from build123d import *

# Parameters (mm, degrees)
F0_R     = 17
F0_R_2   = 1.5
F0_R_3   = 1
F1_DEPTH = 15
F2_START = 10
F2_DEPTH = 15
F3_DEPTH = 5


# Not quite as in the source:
# - a feature names something its author has since deleted; it is built from what else it names


with BuildPart() as f1:
    # F0 (on Front) → F1 (new body)
    with BuildSketch(Plane.XZ):
        Circle(F0_R)
        with BuildLine():
            ThreePointArc((-4.2152867015, -5.2422664968), (-4.1715341961, -5.447511614), (-4.1568542495, -5.6568542495))
            ThreePointArc((-4.1568542495, -5.6568542495), (-6.8551617286, -6.5591065343), (-5.2422664968, -4.2152867015))
            ThreePointArc((-5.2422664968, -4.2152867015), (-4.2289624147, -3.2427342391), (-3.2426406871, -4.2426406871))
            ThreePointArc((-3.2426406871, -4.2426406871), (-3.525928058, -4.9400093179), (-4.2152867015, -5.2422664968))
        make_face(mode=Mode.SUBTRACT)
        with Locations((6.7175144213, -6.7175144213)):
            Circle(F0_R_2, mode=Mode.SUBTRACT)
        with Locations((4.2426406871, -4.2426406871)):
            Circle(F0_R_3, mode=Mode.SUBTRACT)
        with Locations((-4.2426406871, 4.2426406871)):
            Circle(F0_R_3, mode=Mode.SUBTRACT)
        with Locations((-6.7175144213, 6.7175144213)):
            Circle(F0_R_2, mode=Mode.SUBTRACT)
        with BuildLine():
            ThreePointArc((4.2152867015, 5.2422664968), (5.447511614, 7.1421743029), (7.1568542495, 5.6568542495))
            ThreePointArc((7.1568542495, 5.6568542495), (6.5591065343, 4.4585467704), (5.2422664968, 4.2152867015))
            ThreePointArc((5.2422664968, 4.2152867015), (3.5355339059, 3.5355339059), (4.2152867015, 5.2422664968))
        make_face(mode=Mode.SUBTRACT)
        with BuildLine():
            ThreePointArc((5.2422664968, 4.2152867015), (6.5591065343, 4.4585467704), (7.1568542495, 5.6568542495))
            ThreePointArc((7.1568542495, 5.6568542495), (5.447511614, 7.1421743029), (4.2152867015, 5.2422664968))
            ThreePointArc((4.2152867015, 5.2422664968), (4.9400093179, 4.9593533163), (5.2426406871, 4.2426406871))
            ThreePointArc((5.2426406871, 4.2426406871), (5.2425471352, 4.2289624147), (5.2422664968, 4.2152867015))
        make_face()
        with BuildLine():
            ThreePointArc((5.2422664968, 4.2152867015), (4.5961940777, 4.5961940777), (4.2152867015, 5.2422664968))
            ThreePointArc((4.2152867015, 5.2422664968), (3.5355339059, 3.5355339059), (5.2422664968, 4.2152867015))
        make_face()
        with BuildLine():
            ThreePointArc((-5.2422664968, -4.2152867015), (-6.8551617286, -6.5591065343), (-4.1568542495, -5.6568542495))
            ThreePointArc((-4.1568542495, -5.6568542495), (-4.1715341961, -5.447511614), (-4.2152867015, -5.2422664968))
            ThreePointArc((-4.2152867015, -5.2422664968), (-4.9497474683, -4.9497474683), (-5.2422664968, -4.2152867015))
        make_face()
        with BuildLine():
            ThreePointArc((-5.2422664968, -4.2152867015), (-4.9497474683, -4.9497474683), (-4.2152867015, -5.2422664968))
            ThreePointArc((-4.2152867015, -5.2422664968), (-4.5961940777, -4.5961940777), (-5.2422664968, -4.2152867015))
        make_face()
        with BuildLine():
            ThreePointArc((-5.2422664968, -4.2152867015), (-4.5961940777, -4.5961940777), (-4.2152867015, -5.2422664968))
            ThreePointArc((-4.2152867015, -5.2422664968), (-3.525928058, -4.9400093179), (-3.2426406871, -4.2426406871))
            ThreePointArc((-3.2426406871, -4.2426406871), (-4.2289624147, -3.2427342391), (-5.2422664968, -4.2152867015))
        make_face()
        with BuildLine():
            ThreePointArc((5.2426406871, 4.2426406871), (4.9400093179, 4.9593533163), (4.2152867015, 5.2422664968))
            ThreePointArc((4.2152867015, 5.2422664968), (4.5961940777, 4.5961940777), (5.2422664968, 4.2152867015))
            ThreePointArc((5.2422664968, 4.2152867015), (5.2425471352, 4.2289624147), (5.2426406871, 4.2426406871))
        make_face()
        with Locations((4.2426406871, -4.2426406871)):
            Circle(F0_R_3)
        with Locations((-4.2426406871, 4.2426406871)):
            Circle(F0_R_3)
        with Locations((-6.7175144213, 6.7175144213)):
            Circle(F0_R_2)
        with Locations((6.7175144213, -6.7175144213)):
            Circle(F0_R_2)
    extrude(amount=F1_DEPTH)

    # F0 (on Front) → F2 (cut)
    with BuildSketch(Plane.XZ.offset(F2_START)):
        with BuildLine():
            ThreePointArc((-5.2422664968, -4.2152867015), (-4.5961940777, -4.5961940777), (-4.2152867015, -5.2422664968))
            ThreePointArc((-4.2152867015, -5.2422664968), (-3.525928058, -4.9400093179), (-3.2426406871, -4.2426406871))
            ThreePointArc((-3.2426406871, -4.2426406871), (-4.2289624147, -3.2427342391), (-5.2422664968, -4.2152867015))
        make_face()
        with BuildLine():
            ThreePointArc((-5.2422664968, -4.2152867015), (-4.9497474683, -4.9497474683), (-4.2152867015, -5.2422664968))
            ThreePointArc((-4.2152867015, -5.2422664968), (-4.5961940777, -4.5961940777), (-5.2422664968, -4.2152867015))
        make_face()
        with Locations((4.2426406871, -4.2426406871)):
            Circle(F0_R_3)
        with BuildLine():
            ThreePointArc((5.2422664968, 4.2152867015), (4.5961940777, 4.5961940777), (4.2152867015, 5.2422664968))
            ThreePointArc((4.2152867015, 5.2422664968), (3.5355339059, 3.5355339059), (5.2422664968, 4.2152867015))
        make_face()
        with BuildLine():
            ThreePointArc((5.2426406871, 4.2426406871), (4.9400093179, 4.9593533163), (4.2152867015, 5.2422664968))
            ThreePointArc((4.2152867015, 5.2422664968), (4.5961940777, 4.5961940777), (5.2422664968, 4.2152867015))
            ThreePointArc((5.2422664968, 4.2152867015), (5.2425471352, 4.2289624147), (5.2426406871, 4.2426406871))
        make_face()
        with Locations((-4.2426406871, 4.2426406871)):
            Circle(F0_R_3)
    extrude(amount=F2_DEPTH, mode=Mode.SUBTRACT)

    # F0 (on Front) → F3 (cut)
    with BuildSketch(Plane.XZ):
        with BuildLine():
            ThreePointArc((5.2422664968, 4.2152867015), (6.5591065343, 4.4585467704), (7.1568542495, 5.6568542495))
            ThreePointArc((7.1568542495, 5.6568542495), (5.447511614, 7.1421743029), (4.2152867015, 5.2422664968))
            ThreePointArc((4.2152867015, 5.2422664968), (4.9400093179, 4.9593533163), (5.2426406871, 4.2426406871))
            ThreePointArc((5.2426406871, 4.2426406871), (5.2425471352, 4.2289624147), (5.2422664968, 4.2152867015))
        make_face()
        with BuildLine():
            ThreePointArc((5.2426406871, 4.2426406871), (4.9400093179, 4.9593533163), (4.2152867015, 5.2422664968))
            ThreePointArc((4.2152867015, 5.2422664968), (4.5961940777, 4.5961940777), (5.2422664968, 4.2152867015))
            ThreePointArc((5.2422664968, 4.2152867015), (5.2425471352, 4.2289624147), (5.2426406871, 4.2426406871))
        make_face()
        with BuildLine():
            ThreePointArc((-5.2422664968, -4.2152867015), (-6.8551617286, -6.5591065343), (-4.1568542495, -5.6568542495))
            ThreePointArc((-4.1568542495, -5.6568542495), (-4.1715341961, -5.447511614), (-4.2152867015, -5.2422664968))
            ThreePointArc((-4.2152867015, -5.2422664968), (-4.9497474683, -4.9497474683), (-5.2422664968, -4.2152867015))
        make_face()
        with BuildLine():
            ThreePointArc((-5.2422664968, -4.2152867015), (-4.9497474683, -4.9497474683), (-4.2152867015, -5.2422664968))
            ThreePointArc((-4.2152867015, -5.2422664968), (-4.5961940777, -4.5961940777), (-5.2422664968, -4.2152867015))
        make_face()
        with Locations((6.7175144213, -6.7175144213)):
            Circle(F0_R_2)
        with Locations((-6.7175144213, 6.7175144213)):
            Circle(F0_R_2)
    extrude(amount=F3_DEPTH, mode=Mode.SUBTRACT)


solid = f1.part
Design review of the part built by this model. Coordinates are the model's own, in mm. A direction names the side the tool comes from. Give positions to 0.01 mm unless a question says otherwise; leave off trailing zeros. Order: outer loops, then holes, each group sorted by start corner. A loop starts at its lowest first (then second) coordinate and runs counter-clockwise, first axis right, second up.
1. Add section C-C, the plane x = 10. State the section outline as (y, z) points.
Solution:
outline: (-15, -13.75) - (0, -13.75) - (0, 13.75) - (-15, 13.75) - close
2. Tool access review of faces 1 (the cylindrical face through (-7.908, -2.465, 5.805)), 2 (the cylindrical face through (-5.036, -12.465, 3.634)), 3 (the flat face through (0, 0, 0)): name each direction out of +Z, -Z, +X, -X, +Y, -Y from which nothing blocks a thin tool from reaching the whole face with its end or side.
Solution:
face 1: +Y
face 2: -Y
face 3: +Z, -Z, +X, -X, +Y
3. Add section B-B, the plane y = -7. State the section outline as (x, z) points.
Solution:
outline: circle Ø34 at (0, 0)
4. Mouldability with a two-part tool opening along X and no side actions: class faces 4 (the cylindrical face through (3.506, -12.465, -3.567)), 5 (the flat face through (0, -15, 0)), 6 (the cylindrical face through (9.139, -7.395, 14.334)) as +X half, -X half, draft (parallel to the pull), parting line (faces both ways), or undercut.
Solution:
face 4: undercut
face 5: draft
face 6: parting line
5. For pin 1 Ø1.8 at (x, z) = (-5.66, -5.66) entering from +Y; pin 2 Ø6 at (y, z) = (-6.5, -7) entering from -X; pin 3 Ø2 at (x, y) = (12.5, -10) entering from -Z; pin 4 Ø1.5 at (x, z) = (-13, -13) entering from +Y, all flat-tipped, find the tip position at first contact; note any pin that passes through.
Solution:
pin 1: stops at y = -5
pin 2: stops at x = -16.52
pin 3: stops at z = -12.52
pin 4: passes through
6. Add section A-A, the plane y = -4.25. State the section outline as (x, z) points, then the cut area to 3 significant figures.
Solution:
outline: circle Ø34 at (0, 0); hole circle Ø3 at (-6.72, 6.72); hole circle Ø3 at (-5.66, -5.66); hole circle Ø3 at (5.66, 5.66); hole circle Ø3 at (6.72, -6.72)
area: 880 mm2
7. To check wall thickness, follow L1, parallel to X at y = -12.75, z = 4; L2, parallel to X at y = -1.75, z = 6; L3, parallel to Z at x = 0, y = -13.75. State the ranges of each line that lie inside material, in increasing order.
Solution:
L1: x = -16.52 to -5.21, -3.27 to 3.27, 5.21 to 16.52
L2: x = -15.91 to -8.03, -5.4 to 4.2, 7.12 to 15.91
L3: z = -17 to 17
